Geometry check sheet. Reference: the model listing, model coordinates, mm. A direction names the side the tool comes from. Give positions to 0.01 mm unless a question says otherwise; leave off trailing zeros. Loops run counter-clockwise (first coordinate to the right, second up) from the corner with the lowest first, then second, coordinate; pieces in that order, holes last. Notation, with made-up numbers: (25, 66.25) - (66, 66.25) arc R6 cw to (66, 75.25) - close; hole circle Ø8 at (-11.5, 25.5). An arc over 180 degrees is marked (long way). Write item = value, one per line. Start each with the question number.
from build123d import *

# Parameters (mm, degrees)
F1_DEPTH = 3.175
F2_DEPTH = 330.2
F4_DEPTH = 53.975


with BuildPart() as f1:
    # F0 (on Front) → F1 (new body)
    with BuildSketch(Plane.XZ):
        Polygon((-29.6512916684, 86.36), (-29.6512916684, 0), (230.7157522443, 0), (230.7157522443, 28.4875586579), (-22.317701071, 6.35), (-27.298651769, 63.2825269959), (200.4314562148, 83.2063297881), (200.4314562148, 86.36), align=None)
        Polygon((-22.317701071, 6.35), (230.7157522443, 28.4875586579), (200.4314562148, 83.2063297881), (-27.298651769, 63.2825269959), align=None)
    extrude(amount=-F1_DEPTH)

    # F0 (on Front) → F2 (join)
    with BuildSketch(Plane.XZ):
        Polygon((-29.6512916684, 86.36), (-29.6512916684, 0), (230.7157522443, 0), (230.7157522443, 28.4875586579), (-22.317701071, 6.35), (-27.298651769, 63.2825269959), (200.4314562148, 83.2063297881), (200.4314562148, 86.36), align=None)
    extrude(amount=F2_DEPTH)

    # F3 (on face) → F4 (join)
    with BuildSketch(Plane.XZ.offset(330.2)):
        Polygon((-27.298651769, 63.2825269959), (200.4314562148, 83.2063297881), (200.4314562148, 86.36), (-29.6512916684, 86.36), (-29.6512916684, 0), (230.7157522443, 0), (230.7157522443, 28.4875586579), (-22.317701071, 6.35), align=None)
        Polygon((230.7157522443, 28.4875586579), (200.4314562148, 83.2063297881), (-27.298651769, 63.2825269959), (-22.317701071, 6.35), align=None)
    extrude(amount=F4_DEPTH)


solid = f1.part
1) Release check for a two-part mould opening along X. For faces 1 (the face through (-24.773, -162.789, 34.418)), 2 (the face through (84.972, -162.789, 73.105)), 3 (the face through (99, 3.175, 44)) record: pulls with the +X half, pulls with the -X half, needs draft (parallel to the pull), parting line crosses it, or undercut.
2) Cross-section at D-D on z = 51. Enter the section's corners in (x, y) (3 decimals).
3) Gauge pin test, flat ends, axial feed: P1, Ø1.6, axis at y = -249.5, z = 85.5, coming from the +X side; P2, Ø4, axis at y = -338, z = 73, coming from the +X side. Record the tip position at first contact, or that the pin passes through.
4) Tool access check on faces 4 (the face through (99, -188, 0)), 5 (the face through (105.97, -162.789, 17.574)). Record the directions out of +Z, -Z, +X, -X, +Y, -Y that give a thin tool (end or side, any length) a straight path to the whole face; none if there is none.
5) Cross-section at C-C on x = 89. Enter the section's corners in (y, z) (3 decimals).
6) Material ranges on line 1 along Y through (x, z) = (114.5, 75.5) (3 decimals); line 2 along Z through (x, y) = (185.5, -226.5); line 3 along Z through (x, y) = (91, -325), recorded low to high.
7) Cross-section at B-B on y = -52. Enter the section's corners in (x, z).
8) Cross-section at A-A on z = 18.5. Enter the section's corners in (x, y) (3 decimals).
Checked values:
q1.face_1 = undercut
q1.face_2 = pulls with the +X half
q1.face_3 = needs draft
q2.outline = (-29.651, -384.175) - (218.256, -384.175) - (218.256, -330.2) - (-26.224, -330.2) - (-26.224, 0) - (218.256, 0) - (218.256, 3.175) - (-29.651, 3.175) - close
q3.P1 = 200.43
q3.P2 = 207.19
q4.face_4 = -Z, +X, -X, +Y, -Y
q4.face_5 = none
q5.outline = (-384.175, 0) - (3.175, 0) - (3.175, 86.36) - (-384.175, 86.36) - close; hole (-330.2, 16.089) - (0, 16.089) - (0, 73.457) - (-330.2, 73.457) - close
q6.line_1 = -384.175 to -330.2, 0 to 3.175
q6.line_2 = 0 to 24.53, 81.9 to 86.36
q6.line_3 = 0 to 16.26, 73.63 to 86.36
q7.outline = (-29.65, 0) - (230.72, 0) - (230.72, 28.49) - (-22.32, 6.35) - (-27.3, 63.28) - (200.43, 83.21) - (200.43, 86.36) - (-29.65, 86.36) - close
q8.outline = (-29.651, -384.175) - (230.716, -384.175) - (230.716, 3.175) - (-29.651, 3.175) - close; hole (-23.381, -330.2) - (116.557, -330.2) - (116.557, 0) - (-23.381, 0) - close
